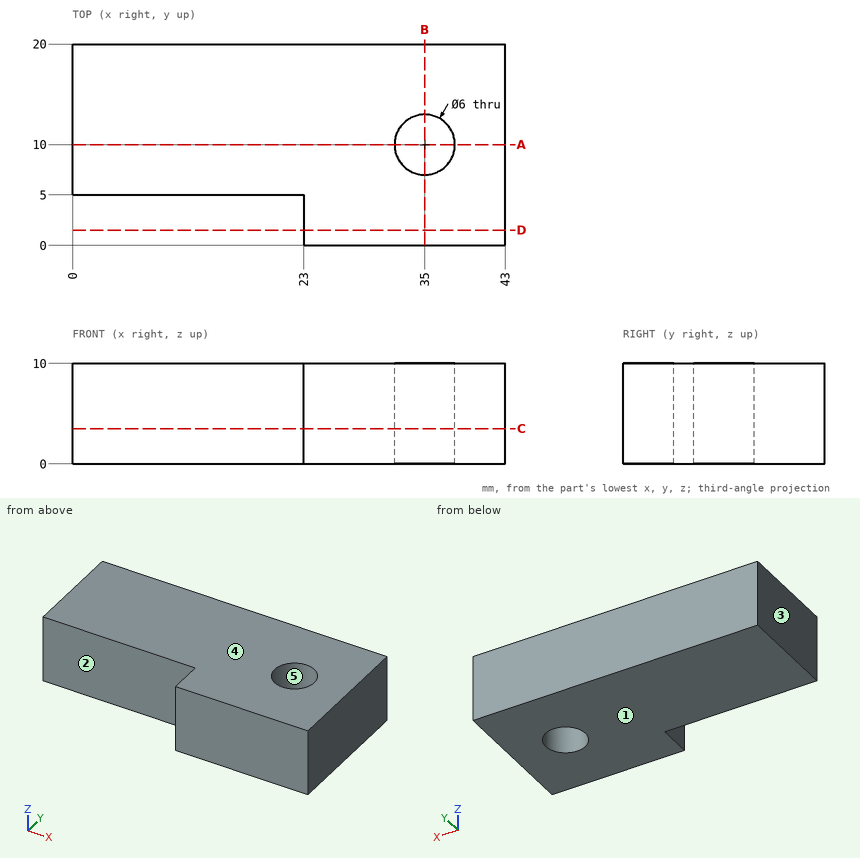
Source: three-view drawing plus pictorial views. Frame: mm from the lowest corner of the part. A direction names the side the tool comes from. Give positions to 0.01 mm unless a question says otherwise; leave off trailing zeros. Loops run counter-clockwise (first coordinate to the right, second up) from the corner with the lowest first, then second, coordinate; pieces in that order, holes last. Notation, with made-up numbers: M 28,70 L 55,70 A20 cw 55,76 Z; hole C 57,-17.5 d5. An arc over 180 degrees is marked long. Put each result on its own line as item: value.
Q1. Section C-C (z = 3.5). Return the cut outline in (x, y), and give its area (3 significant figures).
Response values:
outline: M 0,5 L 23,5 L 23,0 L 43,0 L 43,20 L 0,20 Z; hole C 35,10 d6
area: 717 mm²
Q2. Section D-D (y = 1.5). Return the cut outline in (x, z).
Response values:
outline: M 23,0 L 43,0 L 43,10 L 23,10 Z
Q3. Mould query, pull axis X, two halves, no side actions, for the marked faces 3, 4 and 5. Classes: released by +X, released by -X, zero draft, split by the parting line, or undercut.
Response values:
face 3: released by -X
face 4: zero draft
face 5: undercut
Q4. Pin query (flat end, axial travel): P1, Ø3.5, axis at x = 35, y = 10, coming from the +Z side. Return the tip coordinate at first contact, or that it passes through.
Response values:
P1: passes through
Q5. Reachability of the marked faces 1 and 2 from +Z, -Z, +X, -X, +Y, -Y: full face, straight path, thin tool, end or side. Return the list, or none.
Response values:
face 1: -Z, +X, -X, +Y, -Y
face 2: +Z, -Z, -X, -Y
Q6. Section B-B (x = 35). Return the cut outline in (y, z).
Response values:
outline: M 0,0 L 7,0 L 7,10 L 0,10 Z; M 13,0 L 20,0 L 20,10 L 13,10 Z
Q7. Section A-A (y = 10). Return the cut outline in (x, z).
Response values:
outline: M 0,0 L 32,0 L 32,10 L 0,10 Z; M 38,0 L 43,0 L 43,10 L 38,10 Z
Q8. Line query: probe 1 along Y at (x, z) = (35, 3.5); probe 2 along X at (y, z) = (10, 3.5); probe 3 along X at (y, z) = (3.5, 7.5). Output: solid intervals per line, ascending. Write a range as [from, to].
Response values:
probe 1: y = [0, 7], [13, 20]
probe 2: x = [0, 32], [38, 43]
probe 3: x = [23, 43]
